from build123d import *

# Parameters (mm, degrees)
SKETCH1_R              = 6.35
BOSS_EXTRUDE1_DEPTH    = 53.401902472
CUT_EXTRUDE1_DEPTH     = 55.15171454
F_10_24_TAPPED_HOLE1_D = 3.7973


with BuildPart() as part:
    # Sketch1 → Boss-Extrude1 (new body)
    with BuildSketch(Plane(origin=(0, 0, 0), x_dir=(1, 0, 0), z_dir=(0, 1, 0))):
        with Locations(Location((0, 0, 0), (0, 0, 90))):
            Circle(SKETCH1_R)
    extrude(amount=BOSS_EXTRUDE1_DEPTH)

    # Sketch2 → Cut-Extrude1 (cut, through all)
    with BuildSketch(Plane(origin=(0, 53.401902472, 0), x_dir=(1, 0, 0), z_dir=(0, 1, 0))):
        Polygon((0, -4.445), (-5.65519603, -4.445), (-5.65519603, -6.850474894), (5.907942222, -6.850474894), (5.907942222, -4.445), align=None)
    extrude(amount=-CUT_EXTRUDE1_DEPTH, mode=Mode.SUBTRACT)

    # #10-24 Tapped Hole1 (through all)
    with Locations(Plane.XY.offset(4.445)):
        with Locations((0, 31.988125)):
            Hole(F_10_24_TAPPED_HOLE1_D / 2)


solid = part.part
Read the model definition and answer for the solid it produces. Units are mm, in the model's axes. Give positions to 0.01 mm unless a question says otherwise; leave off trailing zeros. Write each loop counter-clockwise with the first axis right and the second up, starting at its lowest first coordinate (ties: lowest second). Pieces come first, ordered by that corner, then holes. Notation, with made-up numbers: (0.5, 51) - (54.5, 51) arc R26 ccw to (54.5, 75) - close; hole circle Ø2 at (15, 83). An arc over 180 degrees is marked (long way). Use CSV: the item, a comma, the result in double quotes. Start each with the question number.
Item 1: The part is cut by section A-A, the plane x = 0. Give the vertices of the cut face in (y, z) (3 decimals).
Item 2: Consider line 1 (Y direction, x = 0, z = -3.75); line 2 (Y direction, x = -0.5, z = 3.25); line 3 (Z direction, x = -0.5, y = 36.5) (3 decimals). Determine where each line is inside the solid, lowest interval first.
Item 3: The part is cut by section B-B, the plane z = -3. Give the vertices of the cut face in (x, y), and give its area (3 significant figures).
Item 4: A flat-ended cylindrical pin translates along its axis: P1, Ø2, axis at y = 23, z = 3, coming from the -X side. Find the tip coordinate at first contact, or state that the pin passes through.
Item 5: The mould has two halves that part along X. Classify faces 1 (the cylindrical face through (-0.876, 30.304, -1.028)), 2 (the flat face through (0, 27, 4.445)), 3 (the cylindrical face through (0.209, 26.327, -6.347)): pulls with the +X half, pulls with the -X half, needs draft (parallel to the pull), parting line crosses it, or undercut.
Item 6: The part is cut by section C-C, the plane y = 11. Give the vertices of the cut face in (x, z) (3 decimals), and give its area (3 significant figures).
Item 7: The part is cut by section D-D, the plane z = 2.75. Give the vertices of the cut face in (x, y).
Taken from the geometry:
1,outline,"(0, -6.35) - (30.089, -6.35) - (30.089, 4.445) - (0, 4.445) - close; (33.887, -6.35) - (53.402, -6.35) - (53.402, 4.445) - (33.887, 4.445) - close"
2,line 1,"0 to 30.09, 33.89 to 53.4"
2,line 2,"0 to 30.16, 33.82 to 53.4"
2,line 3,"-6.33 to 4.445"
3,outline,"(-5.6, 0) - (5.6, 0) - (5.6, 53.4) - (-5.6, 53.4) - close; hole circle Ø3.8 at (0, 31.99)"
3,area,"586 mm2"
4,P1,"x = -6.03"
5,face 1,"undercut"
5,face 2,"needs draft"
5,face 3,"parting line crosses it"
6,outline,"(-4.535, 4.445) arc R6.35 ccw (long way) to (4.535, 4.445) - close"
6,area,"115 mm2"
7,outline,"(-5.72, 0) - (5.72, 0) - (5.72, 53.4) - (-5.72, 53.4) - close; hole circle Ø3.8 at (0, 31.99)"
